```python
from build123d import *

# Parameters (mm, degrees)
BOSS_EXTRUDE1_DEPTH                   = 3
F_10_0_1935_DIAMETER_HOLE2_AT_2_COUNT = 2
F_10_0_1935_DIAMETER_HOLE2_AT_2_PITCH = 260.668884466
F_10_0_1935_DIAMETER_HOLE1_D          = 4.9149
F_10_0_1935_DIAMETER_HOLE1_DEPTH      = 76.2
F_10_0_1935_DIAMETER_HOLE1_TIP        = 1.476584928
SKETCH9_W                             = 31.5468
SKETCH9_H                             = 5.7658
SKETCH9_W_2                           = 5.7658
SKETCH9_H_2                           = 31.5468
CUT_EXTRUDE1_DEPTH                    = 4


with BuildPart() as part:
    # Sketch1 → Boss-Extrude1 (new body)
    with BuildSketch(Plane.XY):
        with BuildLine():
            Line((-135.866260139, -66.675), (-135.866260139, -314.579))
            Line((-135.866260139, -314.579), (-135.866260139, -371.729))
            ThreePointArc((-135.866260139, -371.729), (-133.07645223, -378.464192091), (-126.341260139, -381.254))
            Line((-126.341260139, -381.254), (261.008739861, -381.254))
            ThreePointArc((261.008739861, -381.254), (267.743931952, -378.464192091), (270.533739861, -371.729))
            Line((270.533739861, -371.729), (270.533739861, -298.704))
            Line((270.533739861, -298.704), (270.533739861, -196.977))
            Line((270.533739861, -196.977), (259.683417693, -196.977))
            ThreePointArc((259.683417693, -196.977), (229.258739861, -190.627), (259.683417693, -184.277))
            Line((259.683417693, -184.277), (270.533739861, -184.277))
            Line((270.533739861, -184.277), (270.533739861, -82.55))
            Line((270.533739861, -82.55), (270.533739861, -9.525))
            ThreePointArc((270.533739861, -9.525), (267.743931952, -2.789807909), (261.008739861, 0))
            Line((261.008739861, 0), (-126.341260139, 0))
            ThreePointArc((-126.341260139, 0), (-133.07645223, -2.789807909), (-135.866260139, -9.525))
            Line((-135.866260139, -9.525), (-135.866260139, -66.675))
        make_face()
    extrude(amount=BOSS_EXTRUDE1_DEPTH)

    # Sketch2 → #10 (0.1935) Diameter Hole3 (revolve, cut)
    with BuildSketch(Plane(origin=(-123.166260139, -12.7, 3), x_dir=(0, -1, 0), z_dir=(1, 0, 0))):
        Polygon((0, 0), (0, 77.676584928), (2.45745, 76.2), (2.45745, 0), align=None)
    f_10_0_1935_diameter_hole3 = revolve(axis=Axis((-123.166260139, -12.7, 9.35), (0, 0, -1)), mode=Mode.SUBTRACT)

    # Sketch7 → #10 (0.1935) Diameter Hole2 (revolve, cut)
    with BuildSketch(Plane(origin=(67.333739861, -12.7, 0), x_dir=(0, 1, 0), z_dir=(1, 0, 0))):
        Polygon((0, 0), (0, 77.676584928), (2.45745, 76.2), (2.45745, 0), align=None)
    f_10_0_1935_diameter_hole2 = revolve(axis=Axis((67.333739861, -12.7, -6.35), (0, 0, 1)), mode=Mode.SUBTRACT)

    # #10 (0.1935) Diameter Hole2 at 2: #10 (0.1935) Diameter Hole2 ×2
    with Locations(*[Vector(-0.730812196, -0.682578591, 0) * (i * F_10_0_1935_DIAMETER_HOLE2_AT_2_PITCH) for i in range(1, F_10_0_1935_DIAMETER_HOLE2_AT_2_COUNT)]):
        add(f_10_0_1935_diameter_hole2, mode=Mode.SUBTRACT)

    # Mirror1: #10 (0.1935) Diameter Hole3 across plane
    add(f_10_0_1935_diameter_hole3.mirror(Plane.ZY.offset(-67.333739861)), mode=Mode.SUBTRACT)

    # Mirror2: #10 (0.1935) Diameter Hole3, #10 (0.1935) Diameter Hole2 across plane
    add(f_10_0_1935_diameter_hole3.mirror(Plane.ZX.offset(-190.627)), mode=Mode.SUBTRACT)
    add(f_10_0_1935_diameter_hole2.mirror(Plane.ZX.offset(-190.627)), mode=Mode.SUBTRACT)

    # Mirror2 copy 1 sketch → Mirror2 copy 1 (revolve, cut)
    with BuildSketch(Plane(origin=(257.833739861, -368.554, 3), x_dir=(0, 1, 0), z_dir=(-1, 0, 0))):
        Polygon((0, 0), (0, 77.676584928), (2.45745, 76.2), (2.45745, 0), align=None)
    revolve(axis=Axis((257.833739861, -368.554, 9.35), (0, 0, -1)), mode=Mode.SUBTRACT)

    # Mirror2 copy 2 sketch → Mirror2 copy 2 (revolve, cut)
    with BuildSketch(Plane(origin=(-123.166260139, -190.627, 0), x_dir=(0, -1, 0), z_dir=(1, 0, 0))):
        Polygon((0, 0), (0, -77.676584928), (2.45745, -76.2), (2.45745, 0), align=None)
    revolve(axis=Axis((-123.166260139, -190.627, -6.35), (0, 0, -1)), mode=Mode.SUBTRACT)

    # #10 (0.1935) Diameter Hole1
    with Locations(Plane(origin=(257.833739861, -241.426988864, 0), x_dir=(-1, 0, 0), z_dir=(0, 0, -1))):
        with Locations((0, 0), (-0.067272713, 101.599977728)):
            Hole(F_10_0_1935_DIAMETER_HOLE1_D / 2, depth=F_10_0_1935_DIAMETER_HOLE1_DEPTH)
            with Locations((0, 0, -(F_10_0_1935_DIAMETER_HOLE1_DEPTH + F_10_0_1935_DIAMETER_HOLE1_TIP / 2))):  # 118° drill point
                Cone(0, F_10_0_1935_DIAMETER_HOLE1_D / 2, F_10_0_1935_DIAMETER_HOLE1_TIP, mode=Mode.SUBTRACT)

    # Sketch9 → Cut-Extrude1 (cut, through all)
    with BuildSketch(Plane(origin=(0, 0, 0), x_dir=(-1, 0, 0), z_dir=(0, 0, -1))):
        with Locations((-121.308739861, -320.675)):
            Rectangle(SKETCH9_W, SKETCH9_H)
        with Locations((-226.083739861, -320.675)):
            Rectangle(SKETCH9_W, SKETCH9_H)
        with Locations((-194.333739861, -285.877)):
            Rectangle(SKETCH9_W_2, SKETCH9_H_2)
        with Locations((-194.333739861, -190.627)):
            Rectangle(SKETCH9_W_2, SKETCH9_H_2)
        with Locations((-194.333739861, -95.377)):
            Rectangle(SKETCH9_W_2, SKETCH9_H_2)
        with Locations((-226.083739861, -60.579)):
            Rectangle(SKETCH9_W, SKETCH9_H)
        with Locations((-121.308739861, -60.579)):
            Rectangle(SKETCH9_W, SKETCH9_H)
        with Locations((-13.358739861, -60.579)):
            Rectangle(SKETCH9_W, SKETCH9_H)
        with Locations((91.416260139, -60.579)):
            Rectangle(SKETCH9_W, SKETCH9_H)
        with Locations((59.932960139, -351.90938)):
            Rectangle(SKETCH9_W_2, SKETCH9_H_2)
        with Locations((59.932960139, -29.34462)):
            Rectangle(SKETCH9_W_2, SKETCH9_H_2)
        with Locations((91.416260139, -320.675)):
            Rectangle(SKETCH9_W, SKETCH9_H)
        with Locations((-13.358739861, -320.675)):
            Rectangle(SKETCH9_W, SKETCH9_H)
    extrude(amount=-CUT_EXTRUDE1_DEPTH, mode=Mode.SUBTRACT)


solid = part.part
```
Model file for the job. Use its own axes, mm. Round coordinates to 2 decimals unless told otherwise and drop trailing zeros. Answer as CSV lines item,"result".
1. Mould opens along Y. For faces 1 (the face through (229.27, -191.23, 1.48)), 2 (the face through (-133.15, -378.39, 1.48)), 3 (the face through (64, -188, 0)), 4 (the face through (267.818, -2.864, 1.479)) say: +Y half, -Y half, draft (parallel to the pull), parting line (faces both ways), or undercut.
Resolved:
face 1,"undercut"
face 2,"-Y half"
face 3,"draft"
face 4,"+Y half"
2. Drill centre lines: line 1 (Y direction, x = 222.5, z = 2); line 2 (X direction, y = -12.7, z = 0.8); line 3 (X direction, y = -295, z = 2.6). Where is each one in solid material? Low to high.
Resolved:
line 1,"-381.25 to -323.56, -317.79 to -63.46, -57.7 to 0"
line 2,"-135.87 to -125.62, -120.71 to 64.88, 69.79 to 255.38, 260.29 to 270.53"
line 3,"-135.87 to 191.45, 197.22 to 270.53"
3. Slice it at A-A, the plane z = 2.1. State how many separate pieces and enclosed holes the cut face has, plus the area to 3 significant figures.
Resolved:
separate pieces,"1"
enclosed holes,"22"
area,"151,000 mm²"
4. Pin check, flat tip, straight feed: pin 1 Ø3 at (x, y) = (-123.17, -190.63) entering from -Z. Stop position of the tip, or through.
Resolved:
pin 1,"through"
